Part model, mm, in its own coordinate system. Round coordinates to 2 decimals unless told otherwise and drop trailing zeros. Write each loop counter-clockwise with the first axis right and the second up, starting at its lowest first coordinate (ties: lowest second). Pieces come first, ordered by that corner, then holes. Notation, with made-up numbers: (8.25, 13) -> (46.25, 13) arc R13 cw to (46.25, 36) -> close; hole circle Ø11 at (84.5, 33). An arc over 180 degrees is marked (long way). Use CSV: the item, a comma, the result in double quotes. Start each with the question number.
(1) Probe line 1 (X direction, y = -8.5, z = 0.4); line 2 (X direction, y = 9, z = 0.6); line 3 (Y direction, x = 0, z = 2.2). List the from-to ranges inside material, lowest first. Write a range as [from, to].
(2) Drop flat-ended pins along their axis: pin 1 (1.5 mm diameter, centred on y = 1.5, z = 2, fed in from -X); pin 2 (1.5 mm diameter, centred on y = -1.5, z = 0.5, fed in from +X). Give the stop position or say it passes through.
(3) Two-plate mould, pull along X, no slides. Class faces 1 (the cylindrical face through (-1.38, -6.2, 1.57)), 2 (the flat face through (-25.586, -29.865, 1.565)), 3 (the flat face through (-457.014, 29.865, 1.565)): released by +X, released by -X, zero draft, split by the parting line, or undercut.
(4) Saw through at B-B (z = 1.4). Count the separate pieces of the cut face and the enclosed holes in it, plus the area to 3 significant figures.
(5) Saw through at A-A (x = -50.8). Give the cut face in (y, z) (3 decimals), plus the area to 3 significant figures.
```python
from build123d import *

# Parameters (mm, degrees)
F0_R     = 1.7272
F0_R_2   = 3.96875
F0_R_3   = 8.221183
F0_R_4   = 6.35
F1_DEPTH = 3.175


with BuildPart() as f1:
    # F0 (on Top) → F1 (new body)
    with BuildSketch(Plane.XY):
        with BuildLine():
            Line((-426.540354, 38.03015), (-488.352253, 21.467701))
            ThreePointArc((-488.352253, 21.467701), (-504.825, 0), (-488.352253, -21.467701))
            Line((-488.352253, -21.467701), (-426.540354, -38.03015))
            Line((-426.540354, -38.03015), (-420.190354, -38.03015))
            Line((-420.190354, -38.03015), (-62.409646, -38.03015))
            Line((-62.409646, -38.03015), (-56.059646, -38.03015))
            Line((-56.059646, -38.03015), (5.752253, -21.467701))
            ThreePointArc((5.752253, -21.467701), (22.225, 0), (5.752253, 21.467701))
            Line((5.752253, 21.467701), (-56.059646, 38.03015))
            Line((-56.059646, 38.03015), (-62.409646, 38.03015))
            Line((-62.409646, 38.03015), (-420.190354, 38.03015))
            Line((-420.190354, 38.03015), (-426.540354, 38.03015))
        make_face()
        with Locations((-405.902854, -30.09265)):
            Circle(F0_R, mode=Mode.SUBTRACT)
        with Locations((-494.386586, -11.786586)):
            Circle(F0_R, mode=Mode.SUBTRACT)
        with Locations((-470.813414, -11.786586)):
            Circle(F0_R_2, mode=Mode.SUBTRACT)
        with Locations((-76.697146, -30.09265)):
            Circle(F0_R, mode=Mode.SUBTRACT)
        with Locations((-11.786586, -11.786586)):
            Circle(F0_R, mode=Mode.SUBTRACT)
        with Locations((11.786586, -11.786586)):
            Circle(F0_R_2, mode=Mode.SUBTRACT)
        with Locations((-482.6, 0)):
            Circle(F0_R_2, mode=Mode.SUBTRACT)
        with Locations((-494.386586, 11.786586)):
            Circle(F0_R_2, mode=Mode.SUBTRACT)
        with Locations((-470.813414, 11.786586)):
            Circle(F0_R, mode=Mode.SUBTRACT)
        with Locations((-405.902854, 30.09265)):
            Circle(F0_R, mode=Mode.SUBTRACT)
        with Locations((-50.8, 0)):
            Circle(F0_R_3, mode=Mode.SUBTRACT)
        Circle(F0_R_4, mode=Mode.SUBTRACT)
        with Locations((-11.786586, 11.786586)):
            Circle(F0_R_2, mode=Mode.SUBTRACT)
        with Locations((11.786586, 11.786586)):
            Circle(F0_R, mode=Mode.SUBTRACT)
        with Locations((-76.697146, 30.09265)):
            Circle(F0_R, mode=Mode.SUBTRACT)
    extrude(amount=F1_DEPTH)


solid = f1.part
```
Answers:
1,line 1,"x = [-503.14, -473.04], [-468.59, 9.56], [14.01, 20.54]"
1,line 2,"x = [-502.92, -497.21], [-491.56, -14.61], [-8.96, 20.32]"
1,line 3,"y = [-23.01, -6.35], [6.35, 23.01]"
2,pin 1,"stops at x = -504.81"
2,pin 2,"stops at x = 22.21"
3,face 1,"undercut"
3,face 2,"released by +X"
3,face 3,"released by -X"
4,separate pieces,"1"
4,enclosed holes,"15"
4,area,"35,900 mm²"
5,outline,"(-36.621, 0) -> (-8.221, 0) -> (-8.221, 3.175) -> (-36.621, 3.175) -> close; (8.221, 0) -> (36.621, 0) -> (36.621, 3.175) -> (8.221, 3.175) -> close"
5,area,"180 mm²"
